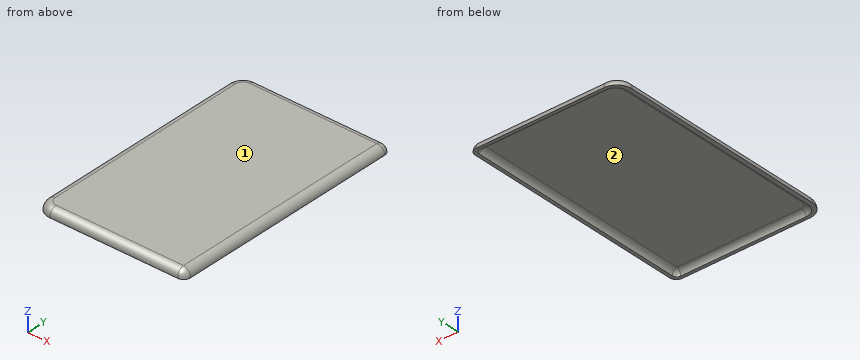
from build123d import *

# Parameters (mm, degrees)
BOX020_W     = 95
BOX020_H     = 155
BOX020_DEPTH = 5.1
FILLET016_R  = 3
FILLET017_R  = 8
FILLET018_R  = 4
BOX019_W     = 100
BOX019_H     = 159
BOX019_DEPTH = 5.1
FILLET012_R  = 10
FILLET013_R  = 4.5
FILLET014_R  = 5


with BuildPart() as fillet018:
    # Box020 → Box020 (new body)
    with BuildSketch(Plane(origin=(23, 7.5, 122.5), x_dir=(1, 0, 0), z_dir=(0, 0, 1))):
        with Locations((47.5, 77.5)):
            Rectangle(BOX020_W, BOX020_H)
    extrude(amount=BOX020_DEPTH)

    # Fillet016
    fillet016_edges = [fillet018.edges().sort_by_distance(p)[0] for p in [
        (118, 7.5, 125.05),
        (118, 162.5, 125.05),
    ]]
    fillet(fillet016_edges, radius=FILLET016_R)

    # Fillet017
    fillet017_edges = [fillet018.edges().sort_by_distance(p)[0] for p in [
        (23, 162.5, 125.05),
        (23, 7.5, 125.05),
    ]]
    fillet(fillet017_edges, radius=FILLET017_R)

    # Fillet018
    fillet018_edges = [fillet018.edges().sort_by_distance(p)[0] for p in [
        (23, 85, 127.6),
    ]]
    fillet(fillet018_edges, radius=FILLET018_R)


with BuildPart() as fillet018_1:
    # Fillet018 placement: moved
    add(fillet018.part.moved(Location((0, 0, -4))))


with BuildPart() as cut354:
    # Box019 → Box019 (new body)
    with BuildSketch(Plane(origin=(19.5, 5.5, 122.5), x_dir=(1, 0, 0), z_dir=(0, 0, 1))):
        with Locations((50, 79.5)):
            Rectangle(BOX019_W, BOX019_H)
    extrude(amount=BOX019_DEPTH)

    # Fillet012
    fillet012_edges = [cut354.edges().sort_by_distance(p)[0] for p in [
        (19.5, 5.5, 125.05),
        (19.5, 164.5, 125.05),
    ]]
    fillet(fillet012_edges, radius=FILLET012_R)

    # Fillet013
    fillet013_edges = [cut354.edges().sort_by_distance(p)[0] for p in [
        (119.5, 5.5, 125.05),
        (119.5, 164.5, 125.05),
    ]]
    fillet(fillet013_edges, radius=FILLET013_R)

    # Fillet014
    fillet014_edges = [cut354.edges().sort_by_distance(p)[0] for p in [
        (72.25, 5.5, 127.6),
        (119.5, 85, 127.6),
        (19.5, 85, 127.6),
        (72.25, 164.5, 127.6),
    ]]
    fillet(fillet014_edges, radius=FILLET014_R)


with BuildPart() as cut354_1:
    # Fillet014 placement: moved
    add(cut354.part.moved(Location((0.7, 0, -2))))

    # Cut014: cut Fillet018
    add(fillet018_1.part, mode=Mode.SUBTRACT)


solid = cut354_1.part
Input: part model. Units: mm. Frame: model coordinates. Face numbers are marked on the shaded views. Coordinates: 2 decimals unless noted, no trailing zeros. Loops run counter-clockwise (first coordinate to the right, second up) from the corner with the lowest first, then second, coordinate; pieces in that order, holes last. Notation, with made-up numbers: (55, 62) -> (114, 62) arc R21 ccw to (114, 89) -> close; hole circle Ø2 at (81, 33). An arc over 180 degrees is marked (long way). Write each question's results on one line, items separated by ' | '. Start each with the question number.
Q1. Pin query (flat end, axial travel): pin 1 (5 mm diameter, centred on x = 67.5, y = 52, fed in from -Z); pin 2 (1 mm diameter, centred on x = 31, z = 121.5, fed in from +Y); pin 3 (1 mm diameter, centred on y = 56.5, z = 123, fed in from -X). Return the tip coordinate at first contact, or that it passes through.
Q2. Section A-A, the plane y = 22. Return the cut outline in (x, z).
Q3. Section B-B, the plane x = 104. Return the cut outline in (y, z), plus the area to 3 significant figures.
Q4. Ray query, line 1 (X direction, y = 25, z = 121.2); line 2 (Z direction, x = 105.5, y = 37); line 3 (X direction, y = 113, z = 123.1). Return the intervals inside material, ascending. Write a range as from..to.
Q5. Pull-direction query (Y, two-part tool) for the marked faces 1 and 2; classes: released by +Y, released by -Y, zero draft, split by the parting line, or undercut.
Found:
1) pin 1: z = 123.6 | pin 2: y = 164.48 | pin 3: x = 20.58
2) outline: (20.2, 120.5) -> (23.1, 120.5) arc R4 cw to (27, 123.6) -> (114, 123.6) arc R4 cw to (117.9, 120.5) -> (120.2, 120.5) -> (120.2, 120.6) arc R5 ccw to (115.2, 125.6) -> (25.2, 125.6) arc R5 ccw to (20.2, 120.6) -> close
3) outline: (5.5, 120.5) -> (7.6, 120.5) arc R4 cw to (11.5, 123.6) -> (158.5, 123.6) arc R4 cw to (162.4, 120.5) -> (164.5, 120.5) -> (164.5, 120.6) arc R5 ccw to (159.5, 125.6) -> (10.5, 125.6) arc R5 ccw to (5.5, 120.6) -> close | area: 326 mm2
4) line 1: 20.24..23.33, 117.67..120.16 | line 2: 123.6..125.6 | line 3: 20.87..25.06, 115.94..119.53
5) face 1: zero draft | face 2: undercut
